Here's how the part is built. I have some questions about the finished solid (model axes, mm). A direction names the side the tool comes from. Round coordinates to 2 decimals unless told otherwise and drop trailing zeros. Order: outer loops, then holes, each group sorted by start corner. A loop starts at its lowest first (then second) coordinate and runs counter-clockwise, first axis right, second up.
```python
from build123d import *

# Parameters (mm, degrees)
SKETCH1_W           = 45.9232
SKETCH1_H           = 21.1074
SKETCH1_R           = 8.0645
BOSS_EXTRUDE1_DEPTH = 6.35
SKETCH2_W           = 4.2418
SKETCH2_H           = 3.429
SKETCH2_W_2         = 12.7
SKETCH2_H_2         = 4.572
CUT_EXTRUDE1_DEPTH  = 6.35
SKETCH4_W           = 5.715
SKETCH4_H           = 3.175
BOSS_EXTRUDE3_DEPTH = 6.35
FILLET1_R           = 1.27


with BuildPart() as part:
    # Sketch1 → Boss-Extrude1 (new body)
    with BuildSketch(Plane(origin=(0, 0, 0), x_dir=(1, 0, 0), z_dir=(0, 1, 0))):
        Rectangle(SKETCH1_W, SKETCH1_H)
        with Locations((-12.6619, 0)):
            Circle(SKETCH1_R, mode=Mode.SUBTRACT)
        with Locations((12.6619, 0)):
            Circle(SKETCH1_R, mode=Mode.SUBTRACT)
    extrude(amount=BOSS_EXTRUDE1_DEPTH)

    # Sketch2 → Cut-Extrude1 (cut)
    with BuildSketch(Plane(origin=(0, 6.35, 0), x_dir=(1, 0, 0), z_dir=(0, 1, 0))):
        with Locations((0, 6.096)):
            Rectangle(SKETCH2_W, SKETCH2_H)
        with Locations((0, -8.2677)):
            Rectangle(SKETCH2_W_2, SKETCH2_H_2)
    extrude(amount=-CUT_EXTRUDE1_DEPTH, mode=Mode.SUBTRACT)

    # Sketch4 → Boss-Extrude3 (add)
    with BuildSketch(Plane(origin=(0, 6.35, 0), x_dir=(1, 0, 0), z_dir=(0, 1, 0))):
        with Locations((-13.7541, -12.1412)):
            Rectangle(SKETCH4_W, SKETCH4_H)
        with Locations((13.7541, -12.1412)):
            Rectangle(SKETCH4_W, SKETCH4_H)
    extrude(amount=-BOSS_EXTRUDE3_DEPTH)

    # Fillet1
    fillet1_edges = [part.edges().sort_by_distance(p)[0] for p in [
        (-6.35, 3.175, 10.5537),
        (-6.35, 3.175, 5.9817),
        (6.35, 3.175, 5.9817),
        (6.35, 3.175, 10.5537),
    ]]
    fillet(fillet1_edges, radius=FILLET1_R)


solid = part.part
```
1) If we section it at B-B (x = 0.5): Write out the boundary of the cut face in (y, z), plus the area to 3 significant figures.
2) We'd pull the mould along Z, two halves only. Please class faces 5 (the cylindrical face through (-5.968, 3.131, 6.344)), 6 (the cylindrical face through (-4.97, 3.13, -2.42)), 7 (the flat face through (0, 0, -1)): +Z half, -Z half, draft (parallel to the pull), parting line (faces both ways), or undercut.
3) If we section it at A-A (z = 0): Write out the boundary of the cut face in (x, y).
4) For faces 1 (the flat face through (6.35, 3, 8)), 2 (the flat face through (20, 3, 10.554)), 3 (the flat face through (-2.121, 3, -6)), 4 (the flat face through (-20, 3, 10.554)), which set-ups out of +Z, -Z, +X, -X, +Y, -Y let a thin tool reach every point of the face, with its end or its side?
5) I'm going to push flat-ended pins straight in: pin 1 (1.9 mm diameter, centred on x = -20.5, y = 2, fed in from +Z); pin 2 (1 mm diameter, centred on y = 4, z = 12, fed in from -X); pin 3 (3.5 mm diameter, centred on y = 4.5, z = 13, fed in from +X); pin 4 (6 mm diameter, centred on x = 16.5, z = -3.5, fed in from -Y). Where does each tip first touch, or does it pass through?
6) If we section it at C-C (y = 1): Write out the boundary of the cut face in (x, z).
7) I need wall thicknesses on line 1 (X direction, y = 2.75, z = 0); line 2 (Z direction, x = -12.5, y = 6.25); line 3 (X direction, y = 3.75, z = -2.25). Which ranges of each line are inside material? Lowest first, please.
8) If we section it at D-D (z = 11.5): Write out the boundary of the cut face in (x, y).
Solutions:
1. outline: (0, -10.55) - (6.35, -10.55) - (6.35, -7.81) - (0, -7.81) - close; (0, -4.38) - (6.35, -4.38) - (6.35, 5.98) - (0, 5.98) - close
1. area: 83.2 mm2
2. face 5: +Z half
2. face 6: undercut
2. face 7: draft
3. outline: (-22.96, 0) - (-20.73, 0) - (-20.73, 6.35) - (-22.96, 6.35) - close; (-4.6, 0) - (4.6, 0) - (4.6, 6.35) - (-4.6, 6.35) - close; (20.73, 0) - (22.96, 0) - (22.96, 6.35) - (20.73, 6.35) - close
4. face 1: +Z, +Y, -Y
4. face 2: +Z, +X, +Y, -Y
4. face 3: +Y, -Y
4. face 4: +Z, -X, +Y, -Y
5. pin 1: stops at z = 10.55
5. pin 2: stops at x = -16.61
5. pin 3: stops at x = 16.61
5. pin 4: stops at y = 0
6. outline: (-22.96, -10.55) - (22.96, -10.55) - (22.96, 10.55) - (16.61, 10.55) - (16.61, 13.73) - (10.9, 13.73) - (10.9, 10.55) - (7.62, 10.55) arc R1.27 ccw to (6.35, 9.28) - (6.35, 7.25) arc R1.27 cw to (5.08, 5.98) - (-5.08, 5.98) arc R1.27 cw to (-6.35, 7.25) - (-6.35, 9.28) arc R1.27 ccw to (-7.62, 10.55) - (-10.9, 10.55) - (-10.9, 13.73) - (-16.61, 13.73) - (-16.61, 10.55) - (-22.96, 10.55) - close; hole circle Ø16.13 at (-12.66, 0); hole (-2.12, -7.81) - (2.12, -7.81) - (2.12, -4.38) - (-2.12, -4.38) - close; hole circle Ø16.13 at (12.66, 0)
7. line 1: x = -22.96 to -20.73, -4.6 to 4.6, 20.73 to 22.96
7. line 2: z = -10.55 to -8.06, 8.06 to 13.73
7. line 3: x = -22.96 to -20.41, -4.92 to 4.92, 20.41 to 22.96
8. outline: (-16.61, 0) - (-10.9, 0) - (-10.9, 6.35) - (-16.61, 6.35) - close; (10.9, 0) - (16.61, 0) - (16.61, 6.35) - (10.9, 6.35) - close
